Could you check a few things on this drawing? It's one solid part, dimensions in mm from its lowest x, y, z. Give positions to 0.01 mm unless a question says otherwise; leave off trailing zeros. Loops run counter-clockwise (first coordinate to the right, second up) from the corner with the lowest first, then second, coordinate; pieces in that order, holes last. Notation, with made-up numbers: (21.5, 38.25) - (65.5, 38.25) arc R23 cw to (65.5, 71.25) - close; hole circle Ø11 at (-24.75, 89). An arc over 180 degrees is marked (long way). Use a Markdown table: item, result.
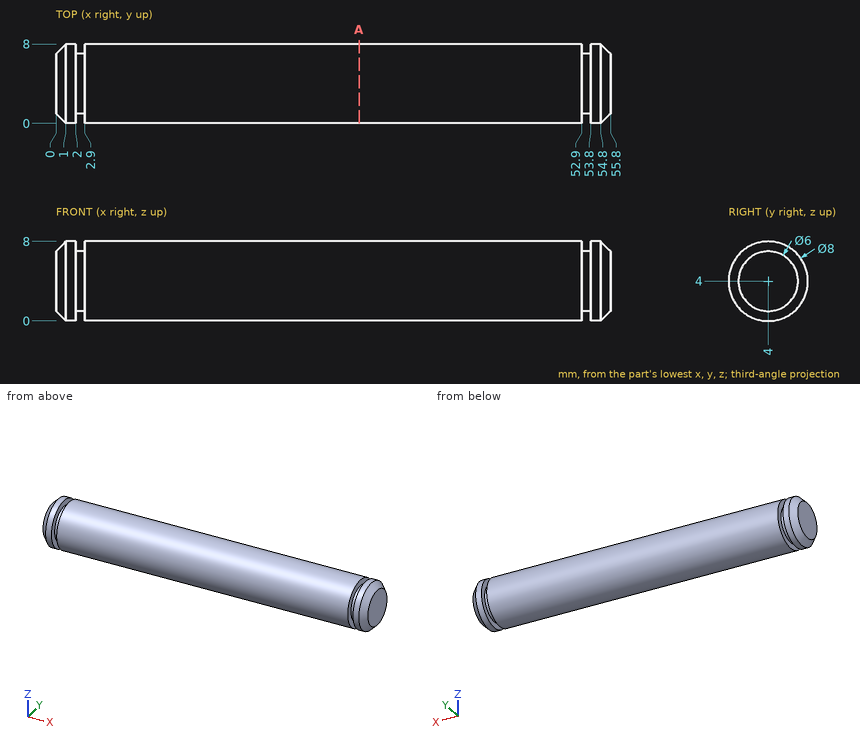
(1) If I drill on line 1 (X direction, y = 1, z = 3); line 2 (X direction, y = 7.5, z = 2.5); line 3 (Z direction, x = 46.5, y = 3.75), over which ranges is the centre line in solid material (lowest first)?
A:
| item | result |
|---|---|
| line 1 | 0.16 to 2, 2.9 to 52.9, 53.8 to 55.64 |
| line 2 | 0.81 to 2, 2.9 to 52.9, 53.8 to 54.99 |
| line 3 | 0.01 to 7.99 |
(2) Will these pins go through, and if not, where does the flat tip stop? pin 1 (1.5 mm diameter, centred on x = 21.5, y = 2.5, fed in from -Z); pin 2 (1 mm diameter, centred on y = 1, z = 2, fed in from +X).
A:
| item | result |
|---|---|
| pin 1 | z = 0.07 |
| pin 2 | x = 55.69 |
(3) Suppose I cut it at A-A on x = 30.5. Write out the boundary of the cut face in (y, z), plus the area to 3 significant figures.
A:
| item | result |
|---|---|
| outline | circle Ø8 at (4, 4) |
| area | 50.3 mm2 |
